The listing builds one solid part. Answer for the finished solid, in the listing's coordinates (mm). A direction names the side the tool comes from. Coordinates: 2 decimals unless noted, no trailing zeros. Order: outer loops, then holes, each group sorted by start corner. A loop starts at its lowest first (then second) coordinate and runs counter-clockwise, first axis right, second up. Notation, with made-up numbers: (-37.75, 3) -> (1.25, 3) arc R28 cw to (1.25, 37) -> close; hole circle Ø10 at (60.25, -16.75). An arc over 180 degrees is marked (long way). Return JSON: item names as keys, results as strings.
from build123d import *

# Parameters (mm, degrees)
SKETCH_1_W             = 18
SKETCH_1_H             = 11
EXTRUDE_1_DEPTH        = 12.5
SKETCH_2_W             = 20.5
SKETCH_2_H             = 14.5
EXTRUDE_2_DEPTH        = 1.5
SKETCH_3_W             = 0.5
SKETCH_3_H             = 7.5
CUT_EXTRUDE_2_DEPTH    = 14.5
EXTRUDE_3_DEPTH        = 1.25
MIRROR_2_COPY_1_DEPTH  = 1.25
SKETCH_7_W             = 18
SKETCH_7_H             = 12.5
EXTRUDE_4_DEPTH        = 2
SKETCH_8_W             = 15
SKETCH_8_H             = 10
CUT_EXTRUDE_3_DEPTH    = 1
EXTRUDE_5_DEPTH        = 4.75
EXTRUDE_5_DEPTH_BACK   = 4.75
SKETCH_11_R            = 0.5
EXTRUDE_6_DEPTH        = 0.75
PATTERN_LINEAR_1_COUNT = 3
PATTERN_LINEAR_1_PITCH = 7


with BuildPart() as part:
    # Эскиз1 → Бобышка-Вытянуть1 (new body)
    with BuildSketch(Plane.XY):
        with Locations((9, 5.5)):
            Rectangle(SKETCH_1_W, SKETCH_1_H)
    extrude(amount=EXTRUDE_1_DEPTH)

    # Эскиз2 → Бобышка-Вытянуть2 (add)
    with BuildSketch(Plane(origin=(0, 11, 0), x_dir=(1, 0, 0), z_dir=(0, 1, 0))):
        with Locations((9, -6.25)):
            Rectangle(SKETCH_2_W, SKETCH_2_H)
    extrude(amount=EXTRUDE_2_DEPTH)

    # Эскиз3 → Вырез-Вытянуть2 (cut, through all)
    with BuildSketch(Plane.XY.offset(12.5)):
        with Locations((17.75, 7.25)):
            Rectangle(SKETCH_3_W, SKETCH_3_H)
        with Locations((0.25, 7.25)):
            Rectangle(SKETCH_3_W, SKETCH_3_H)
    extrude(amount=-CUT_EXTRUDE_2_DEPTH, mode=Mode.SUBTRACT)

    # Эскиз4 → Бобышка-Вытянуть3 (add)
    with BuildSketch(Plane(origin=(17.5, 0, 0), x_dir=(0, 0, -1), z_dir=(1, 0, 0))):
        Polygon((-12.5, 7), (-13, 7.5), (-13, 11), (-12.5, 11), align=None)
    extrude_3 = extrude(amount=-EXTRUDE_3_DEPTH)

    # Зеркальное отражение1: Бобышка-Вытянуть3 across plane
    add(extrude_3.mirror(Plane(origin=(0, 0, 6.25), x_dir=(1, 0, 0), z_dir=(0, 0, -1))))

    # Зеркальное отражение2: Бобышка-Вытянуть3 across plane
    add(extrude_3.mirror(Plane.ZY.offset(-9)))

    # Зеркальное отражение2 copy 1 sketch → Зеркальное отражение2 copy 1 (add)
    with BuildSketch(Plane(origin=(0.5, 0, 12.5), x_dir=(0, 0, 1), z_dir=(-1, 0, 0))):
        Polygon((-12.5, 7), (-13, 7.5), (-13, 11), (-12.5, 11), align=None)
    extrude(amount=-MIRROR_2_COPY_1_DEPTH)

    # Эскиз7 → Бобышка-Вытянуть4 (add)
    with BuildSketch(Plane.XZ):
        with Locations((9, 6.25)):
            Rectangle(SKETCH_7_W, SKETCH_7_H)
    extrude(amount=EXTRUDE_4_DEPTH)

    # Эскиз8 → Вырез-Вытянуть3 (cut)
    with BuildSketch(Plane(origin=(0, 12.5, 0), x_dir=(1, 0, 0), z_dir=(0, 1, 0))):
        with Locations((9, -6.25)):
            Rectangle(SKETCH_8_W, SKETCH_8_H)
    extrude(amount=-CUT_EXTRUDE_3_DEPTH, mode=Mode.SUBTRACT)

    # Эскиз9 → Бобышка-Вытянуть5 (add, two sides)
    with BuildSketch(Plane.YX.offset(-6.25)) as extrude_5_sk:
        with BuildLine():
            Line((11.5, 1.75), (11.5, 16.25))
            ThreePointArc((11.5, 16.25), (12.885675396, 10.16586822), (15.5, 4.5))
            ThreePointArc((15.5, 4.5), (13.669392877, 2.87861036), (11.5, 1.75))
        make_face()
    extrude(amount=EXTRUDE_5_DEPTH)
    extrude(extrude_5_sk.sketch, amount=-EXTRUDE_5_DEPTH_BACK)

    # Эскиз11 → Бобышка-Вытянуть6 (add)
    with BuildSketch(Plane(origin=(1.5, 0, 0), x_dir=(0, 0, 1), z_dir=(1, 0, 0))):
        with BuildLine():
            Line((5.5, 2), (5.5, 7.25))
            ThreePointArc((5.5, 7.25), (5.719669914, 7.780330086), (6.25, 8))
            ThreePointArc((6.25, 8), (6.780330086, 7.780330086), (7, 7.25))
            Line((7, 7.25), (7, 2))
            Line((7, 2), (5.5, 2))
        make_face()
        with Locations((6.25, 7)):
            Circle(SKETCH_11_R, mode=Mode.SUBTRACT)
    extrude_6 = extrude(amount=EXTRUDE_6_DEPTH)

    # Линейный массив1: Бобышка-Вытянуть6 ×3
    with Locations(*[(i * PATTERN_LINEAR_1_PITCH, 0, 0) for i in range(1, PATTERN_LINEAR_1_COUNT)]):
        add(extrude_6)


solid = part.part
1. Determine the mould class of faces 4 (the face through (17, 9, -0.5)), 5 (the face through (15.87, -6.512, 6.142)), 6 (the face through (2.9, 13.7, 6.2)) for opening direction Y: pulls with the +Y half, pulls with the -Y half, needs draft (parallel to the pull), parting line crosses it, or undercut.
Answer block:
{"face 4": "needs draft", "face 5": "undercut", "face 6": "pulls with the +Y half"}
2. Consider line 1 (Z direction, x = 2.05, y = -7); line 2 (Y direction, x = 3.75, z = 1); line 3 (X direction, y = 4.5, z = 8.25). Determine where each line is inside the solid, lowest interval first. Write a range as from..to.
Answer block:
{"line 1": "z = 5.5..5.75, 6.75..7", "line 2": "y = -2..12.5", "line 3": "x = 0.5..17.5"}
3. For faces 1 (the face through (9, 12, 11.25)), 2 (the face through (18, 1, 6)), 3 (the face through (15.5, -5, 6)), determine the directions among +Z, -Z, +X, -X, +Y, -Y from which every point of the face is accessible in a straight line to the end or side of a thin tool.
Answer block:
{"face 1": "+Y", "face 2": "+Z, -Z, +X, -Y", "face 3": "+Z, -Z, -Y"}
4. The part is cut by section C-C on y = 10.5. Give the vertices of the cut face in (x, z), and give its area (3 significant figures).
Answer block:
{"outline": "(0.5, -0.5) -> (1.75, -0.5) -> (1.75, 0) -> (16.25, 0) -> (16.25, -0.5) -> (17.5, -0.5) -> (17.5, 13) -> (16.25, 13) -> (16.25, 12.5) -> (1.75, 12.5) -> (1.75, 13) -> (0.5, 13) -> close", "area": "215 mm2"}
5. The part is cut by section B-B on z = 4.5. Give the vertices of the cut face in (x, y), and give its area (3 significant figures).
Answer block:
{"outline": "(-1.25, 11) -> (0.5, 11) -> (0.5, 3.5) -> (0, 3.5) -> (0, -2) -> (18, -2) -> (18, 3.5) -> (17.5, 3.5) -> (17.5, 11) -> (19.25, 11) -> (19.25, 12.5) -> (16.5, 12.5) -> (16.5, 11.5) -> (16.25, 11.5) arc R30 cw to (4.5, 15.5) arc R10 ccw to (1.75, 11.5) -> (1.5, 11.5) -> (1.5, 12.5) -> (-1.25, 12.5) -> close", "area": "267 mm2"}
6. The part is cut by section D-D on x = 12.75. Give the vertices of the cut face in (y, z).
Answer block:
{"outline": "(-2, 0) -> (11, 0) -> (11, -1) -> (12.5, -1) -> (12.5, 1.25) -> (11.5, 1.25) -> (11.5, 1.5) -> (12.13, 1.5) -> (12.13, 11) -> (11.5, 11) -> (11.5, 11.25) -> (12.5, 11.25) -> (12.5, 13.5) -> (11, 13.5) -> (11, 12.5) -> (-2, 12.5) -> close"}
7. Each of these flat-tipped pins is pushed along its axis until it touches: pin 1 Ø3 at (x, y) = (14.5, 10) entering from +Z; pin 2 Ø0.8 at (y, z) = (-4, 6) entering from +X; pin 3 Ø5 at (y, z) = (-1.5, 5) entering from +X; pin 4 Ø6.5 at (x, y) = (11.5, 1.5) entering from +Z. Where does it stop, or does it pass through?
Answer block:
{"pin 1": "stops at z = 13.5", "pin 2": "stops at x = 16.25", "pin 3": "stops at x = 18", "pin 4": "stops at z = 12.5"}
8. The part is cut by section A-A on y = -4.25. Give the vertices of the cut face in (x, z).
Answer block:
{"outline": "(1.5, 5.5) -> (2.25, 5.5) -> (2.25, 7) -> (1.5, 7) -> close; (8.5, 5.5) -> (9.25, 5.5) -> (9.25, 7) -> (8.5, 7) -> close; (15.5, 5.5) -> (16.25, 5.5) -> (16.25, 7) -> (15.5, 7) -> close"}
